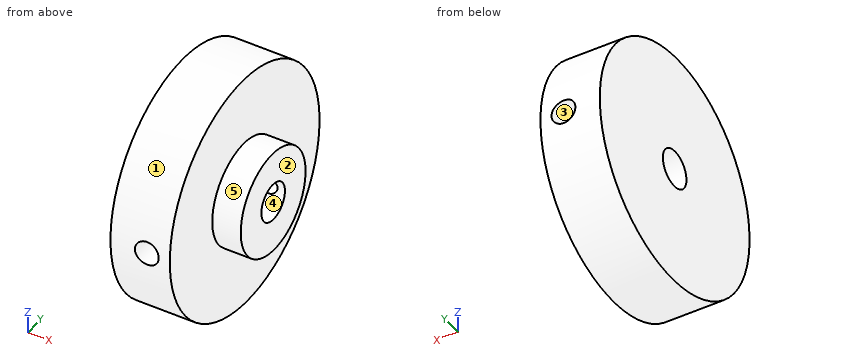
from build123d import *

# Parameters (mm, degrees)
SKETCH2_R                 = 11
BOSS_EXTRUDE2_DEPTH       = 6.1
SKETCH7_R                 = 4
CUT_EXTRUDE3_DEPTH        = 7.1
SKETCH8_R                 = 25.4
BOSS_EXTRUDE3_DEPTH       = 12.7
SKETCH10_R                = 4
CUT_EXTRUDE5_DEPTH        = 13.7
F_1_4_20_TAPPED_HOLE1_D   = 5.1054
M4X0_7_TAPPED_HOLE2_D     = 3.3
M4X0_7_TAPPED_HOLE2_DEPTH = 11.176
M4X0_7_TAPPED_HOLE2_TIP   = 0.991420021


with BuildPart() as part:
    # Sketch2 → Boss-Extrude2 (new body)
    with BuildSketch(Plane(origin=(0, 0, 0), x_dir=(0, 0, -1), z_dir=(1, 0, 0))):
        Circle(SKETCH2_R)
    extrude(amount=BOSS_EXTRUDE2_DEPTH)

    # Sketch7 → Cut-Extrude3 (cut, through all)
    with BuildSketch(Plane(origin=(6.1, 0, 0), x_dir=(0, 0, -1), z_dir=(1, 0, 0))):
        Circle(SKETCH7_R)
    extrude(amount=-CUT_EXTRUDE3_DEPTH, mode=Mode.SUBTRACT)

    # Sketch8 → Boss-Extrude3 (add)
    with BuildSketch(Plane.ZY):
        Circle(SKETCH8_R)
    extrude(amount=BOSS_EXTRUDE3_DEPTH)

    # Sketch10 → Cut-Extrude5 (cut, through all)
    with BuildSketch(Plane(origin=(0, 0, 0), x_dir=(0, 0, -1), z_dir=(1, 0, 0))):
        Circle(SKETCH10_R)
    extrude(amount=-CUT_EXTRUDE5_DEPTH, mode=Mode.SUBTRACT)

    # 1/4-20 Tapped Hole1 (through all)
    with Locations(Plane(origin=(-4.921208149, 25.4, 0), x_dir=(0, 0, 1), z_dir=(0, 1, 0))):
        with Locations((0, 0)):
            Hole(F_1_4_20_TAPPED_HOLE1_D / 2)

    # M4x0.7 Tapped Hole2
    with Locations(Plane(origin=(2.900798662, 11, 0), x_dir=(0, 0, 1), z_dir=(0, 1, 0))):
        with Locations((0, 0)):
            Hole(M4X0_7_TAPPED_HOLE2_D / 2, depth=M4X0_7_TAPPED_HOLE2_DEPTH)
            with Locations((0, 0, -(M4X0_7_TAPPED_HOLE2_DEPTH + M4X0_7_TAPPED_HOLE2_TIP / 2))):  # 118° drill point
                Cone(0, M4X0_7_TAPPED_HOLE2_D / 2, M4X0_7_TAPPED_HOLE2_TIP, mode=Mode.SUBTRACT)


solid = part.part
The model under review builds one solid part; all positions refer to its coordinate system, in mm. Face numbers are marked on the shaded views. A direction names the side the tool comes from. Give positions to 0.01 mm unless a question says otherwise; leave off trailing zeros. Loops run counter-clockwise (first coordinate to the right, second up) from the corner with the lowest first, then second, coordinate; pieces in that order, holes last. Notation, with made-up numbers: (-30.75, 38) -> (15.25, 38) arc R25 cw to (15.25, 72) -> close; hole circle Ø8 at (34, 11). An arc over 180 degrees is marked (long way). Answer as a JSON object with one key per item and string values. Group by question number.
Q1. Take a section at C-C (x = -5.75). Write out the cut boundary in (y, z), plus the area to 3 significant figures.
Q2. Take a section at D-D (z = 8). Write out the cut boundary in (x, y).
Q3. Take a section at B-B (z = 0). Write out the cut boundary in (x, y), plus the area to 3 significant figures.
Q4. Insertion check: pin 1 (5 mm diameter, centred on y = 0, z = 0, fed in from -X); pin 2 (8 mm diameter, centred on x = -7, y = -3, fed in from -Z); pin 3 (4.5 mm diameter, centred on x = 2.9, z = 0, fed in from +Y); pin 4 (2 mm diameter, centred on y = -8.5, z = 14, fed in from +X). Each pin has a flat end and moves straight along its axis. Give the tip position at first contact, or say it passes through.
Q5. Take a section at A-A (y = 0). Write out the cut boundary in (x, z).
Q6. Tool access review of the marked faces 4 and 5: name each direction out of +Z, -Z, +X, -X, +Y, -Y from which nothing blocks a thin tool from reaching the whole face with its end or side.
Q7. Draft analysis for pull direction Z (two halves, no side actions). For the marked faces 1, 2 and 3, state which applies: pulls with the +Z half, pulls with the -Z half, needs draft (parallel to the pull), parting line crosses it, or undercut.
Q8. Wall thickness on line 1 along X through (y, z) = (9, 0); line 2 along X through (y, z) = (-20.5, 0); line 3 along X through (y, z) = (-1.5, -16.5): over which ranges is each line inside the solid? List them lowest first.
Answer below:
{
 "1": {"outline": "(-25.28, -2.41) arc R25.4 ccw to (25.28, -2.41) -> (3.19, -2.41) arc R4 cw to (-3.19, -2.41) -> close; (-25.28, 2.41) -> (-3.19, 2.41) arc R4 cw to (3.19, 2.41) -> (25.28, 2.41) arc R25.4 ccw to start", "area": "1,770 mm2"},
 "2": {"outline": "(-12.7, -24.11) -> (0, -24.11) -> (0, -7.55) -> (6.1, -7.55) -> (6.1, 7.55) -> (0, 7.55) -> (0, 24.11) -> (-12.7, 24.11) -> close"},
 "3": {"outline": "(-12.7, -25.4) -> (-7.47, -25.4) -> (-7.47, -4) -> (-12.7, -4) -> close; (-12.7, 4) -> (-7.47, 4) -> (-7.47, 25.4) -> (-12.7, 25.4) -> close; (-2.37, -25.4) -> (0, -25.4) -> (0, -11) -> (6.1, -11) -> (6.1, -4) -> (-2.37, -4) -> close; (-2.37, 4) -> (1.25, 4) -> (1.25, 11) -> (0, 11) -> (0, 25.4) -> (-2.37, 25.4) -> close; (4.55, 4) -> (6.1, 4) -> (6.1, 11) -> (4.55, 11) -> close", "area": "387 mm2"},
 "4": {"pin 1": "passes through", "pin 2": "stops at z = -25.4", "pin 3": "stops at y = 11", "pin 4": "stops at x = 0"},
 "5": {"outline": "(-12.7, -25.4) -> (0, -25.4) -> (0, -11) -> (6.1, -11) -> (6.1, -4) -> (-12.7, -4) -> close; (-12.7, 4) -> (6.1, 4) -> (6.1, 11) -> (0, 11) -> (0, 25.4) -> (-12.7, 25.4) -> close"},
 "6": {"face 4": "+X, -X", "face 5": "+X"},
 "7": {"face 1": "parting line crosses it", "face 2": "needs draft", "face 3": "undercut"},
 "8": {"line 1": "x = -12.7 to -7.47, -2.37 to 1.25, 4.55 to 6.1", "line 2": "x = -12.7 to -7.47, -2.37 to 0", "line 3": "x = -12.7 to 0"}
}
